For this review, use the dimensioned drawing (mm, ordinates from the lowest corner) and the shaded views. A direction names the side the tool comes from. Coordinates: 2 decimals unless noted, no trailing zeros. Loops run counter-clockwise (first coordinate to the right, second up) from the corner with the lowest first, then second, coordinate; pieces in that order, holes last. Notation, with made-up numbers: (-29.5, -37) - (27.5, -37) arc R36 cw to (27.5, -3) - close; hole circle Ø10 at (54.25, -36.5). An arc over 180 degrees is marked (long way). Answer in a Markdown table with one row per item. Add a question column.
(1) Clearance check with flat-ended pins moving along their axes: pin 1 (4 mm diameter, centred on x = 17.5, z = 10, fed in from -Y); pin 2 (1.5 mm diameter, centred on x = 13, z = 12.5, fed in from -Y). State where each tip first meets the part, or that it passes through.
(2) We need section A-A, the plane y = 3. Write out the cut boundary in (x, z).
(3) To check wall thickness, follow L1, parallel to X at y = 4, z = 20; L2, parallel to Z at x = 2, y = 5.75; L3, parallel to X at y = 1, z = 14.75. State the ranges of each line that lie inside material, in increasing order. Write a range as [from, to].
(4) We need section B-B, the plane x = 2.5. Write out the cut boundary in (y, z), plus the area to 3 significant figures.
(5) For the marked faces 1 and 2, list the 3-axis set-ups (+Z, -Z, +X, -X, +Y, -Y) from which the entire face can be reached by the end or side of a thin tool; tool diameter is ignored.
(6) The part is to be moulded in two halves that separate along X. For the marked faces 3, 4, 5 and 6, say which applies: released by +X, released by -X, zero draft, split by the parting line, or undercut.
(7) We need section D-D, the plane y = 6.5. Write out the cut boundary in (x, z).
(8) We need section C-C, the plane z = 10. Write out the cut boundary in (x, y).
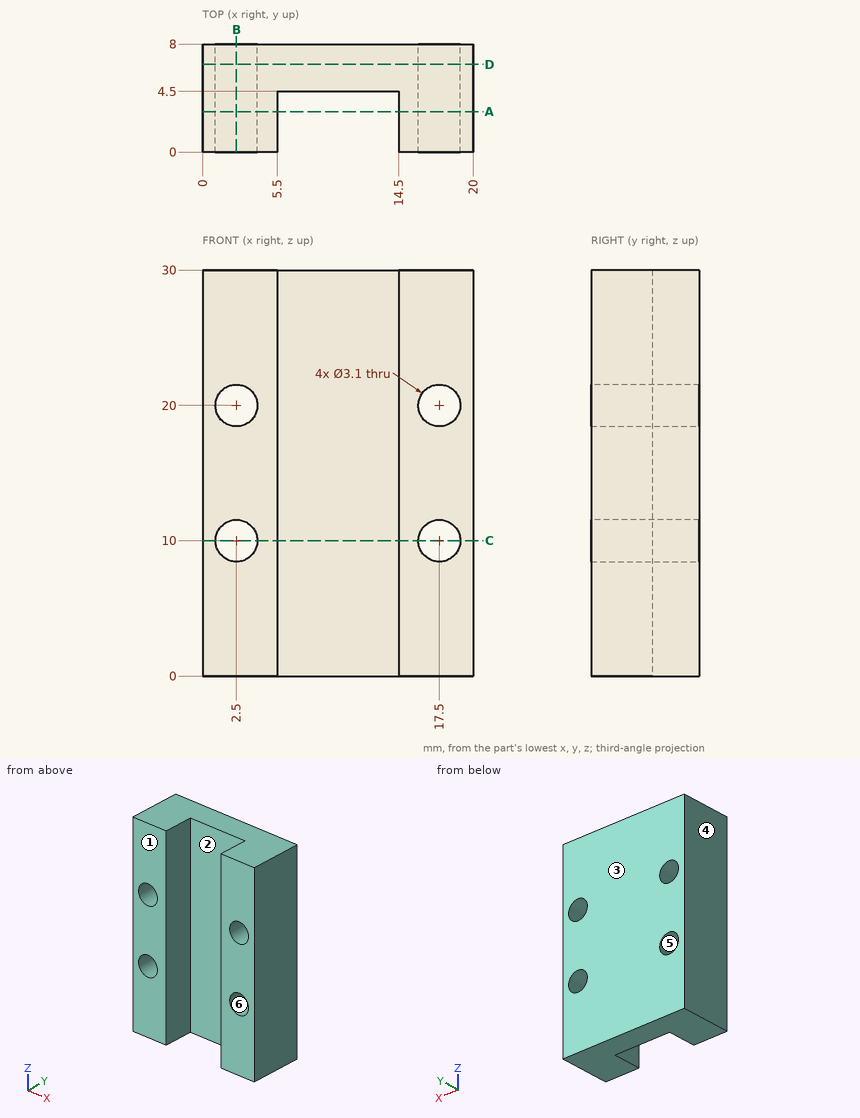
Responses:
| question | item | result |
|---|---|---|
| 1 | pin 1 | stops at y = 0 |
| 1 | pin 2 | stops at y = 4.5 |
| 2 | outline | (0, 0) - (5.5, 0) - (5.5, 30) - (0, 30) - close; (14.5, 0) - (20, 0) - (20, 30) - (14.5, 30) - close; hole circle Ø3.1 at (2.5, 10); hole circle Ø3.1 at (2.5, 20); hole circle Ø3.1 at (17.5, 10); hole circle Ø3.1 at (17.5, 20) |
| 3 | L1 | x = [0, 0.95], [4.05, 5.5], [14.5, 15.95], [19.05, 20] |
| 3 | L2 | z = [0, 8.53], [11.47, 18.53], [21.47, 30] |
| 3 | L3 | x = [0, 5.5], [14.5, 20] |
| 4 | outline | (0, 0) - (8, 0) - (8, 8.45) - (0, 8.45) - close; (0, 11.55) - (8, 11.55) - (8, 18.45) - (0, 18.45) - close; (0, 21.55) - (8, 21.55) - (8, 30) - (0, 30) - close |
| 4 | area | 190 mm2 |
| 5 | face 1 | +Z, -Z, +X, -X, -Y |
| 5 | face 2 | +Z, -Z, -Y |
| 6 | face 3 | zero draft |
| 6 | face 4 | released by -X |
| 6 | face 5 | undercut |
| 6 | face 6 | undercut |
| 7 | outline | (0, 0) - (20, 0) - (20, 30) - (0, 30) - close; hole circle Ø3.1 at (2.5, 10); hole circle Ø3.1 at (2.5, 20); hole circle Ø3.1 at (17.5, 10); hole circle Ø3.1 at (17.5, 20) |
| 8 | outline | (0, 0) - (0.95, 0) - (0.95, 8) - (0, 8) - close; (4.05, 0) - (5.5, 0) - (5.5, 4.5) - (14.5, 4.5) - (14.5, 0) - (15.95, 0) - (15.95, 8) - (4.05, 8) - close; (19.05, 0) - (20, 0) - (20, 8) - (19.05, 8) - close |
